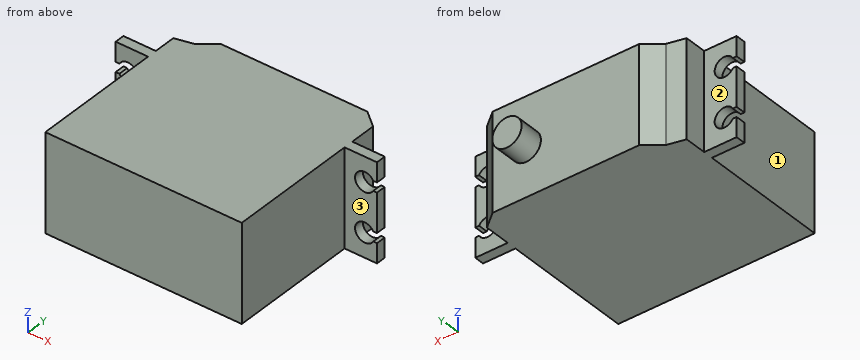
Autodesk Inventor part; units mm, degrees
ref_plane "YZ Plane" through (0, 0, 0) normal (1, 0, 0) x (0, 1, 0)
ref_plane "XZ Plane" through (0, 0, 0) normal (0, 1, 0) x (-1, 0, 0)
ref_plane "XY Plane" through (0, 0, 0) normal (0, 0, 1) x (1, 0, 0)
sketch "Skizze1" plane through (0, 0, 0) normal (0, 0, 1) x (1, 0, 0)
  line L0 (-20.15, 13.3) -> (20.15, 13.3)
  line L1 (20.15, 13.3) -> (20.15, -13.3)
  line L2 (20.15, -13.3) -> (-20.15, -13.3)
  line L3 (-20.15, -13.3) -> (-20.15, 13.3)
  line L4 (0, 30.62) -> (0, -20.62)
  line L5 (-37.52, 0) -> (37.52, 0)
  line L6 (-20.15, 13.3) -> (-20.15, 19.8141)
  line L7 (-13.1284, 23.3) -> (16.9083, 23.3)
  line L8 (20.15, 20.6722) -> (20.15, 13.3)
  line L9 (16.9083, 23.3) -> (20.15, 20.6722)
  line L10 (-20.15, 19.8141) -> (-16.5313, 20.6722)
  line L11 (-16.5313, 20.6722) -> (-13.1284, 23.3)
  line L12 (20.15, 13.3) -> (26.8, 13.3)
  line L13 (26.8, 13.3) -> (26.8, 15.3)
  line L14 (26.8, 15.3) -> (20.15, 15.3)
  line L15 (20.15, 15.3) -> (20.15, 13.3)
  line L16 (-20.15, 13.3) -> (-26.8, 13.3)
  line L17 (-26.8, 13.3) -> (-26.8, 15.3)
  line L18 (-26.8, 15.3) -> (-20.15, 15.3)
  line L19 (-20.15, 15.3) -> (-20.15, 13.3)
  line L20 (6, 23.3) -> (11, 23.3)
  point P0 (0, 0)
  dimension "d0" = 40.3
  dimension "d1" = 26.6
  dimension "d3" = 10
  dimension "d4" = 3.6187
  dimension "d5" = 3.4029
  dimension "d6" = 3.2417
  dimension "d7" = 103.34
  dimension "d8" = 142.325
  dimension "d9" = 140.972
  dimension "d10" = 6.65
  dimension "d11" = 2
  dimension "d12" = 6.65
  dimension "d13" = 2
extrude "Extrusion1" add sketch "Skizze1" along normal mid plane 20
sketch "Skizze2" plane through (-26.8, 15.3, 10) normal (0, 1, 0) x (1, 0, 0)
  line L0 (64.32, 10) -> (-10.72, 10)
  line L1 (26.8, 24) -> (26.8, -4)
  arc A0 (0.7679, 14) -> (0.7679, 16) centre (2.5, 15) ccw
  line L2 (0, 20) -> (0, 0)
  line L3 (0.7679, 16) -> (0, 16)
  line L4 (0, 20) -> (0, 0)
  line L5 (0.7679, 14) -> (0, 14)
  line L6 (0, 16) -> (0, 14)
  line L7 (2.5, 15) -> (0.8619, 15)
  arc A1 (0.7679, 4) -> (0.7679, 6) centre (2.5, 5) ccw
  line L8 (0.7679, 4) -> (0, 4)
  line L9 (0.7679, 6) -> (0, 6)
  line L10 (0, 4) -> (0, 6)
  line L11 (2.5, 5) -> (0.8619, 5)
  arc A2 (52.8321, 16) -> (52.8321, 14) centre (51.1, 15) ccw
  line L12 (52.8321, 16) -> (53.6, 16)
  line L13 (52.8321, 14) -> (53.6, 14)
  line L14 (53.6, 16) -> (53.6, 14)
  line L15 (51.1, 15) -> (52.7381, 15)
  arc A3 (52.8321, 6) -> (52.8321, 4) centre (51.1, 5) ccw
  line L16 (52.8321, 4) -> (53.6, 4)
  line L17 (52.8321, 6) -> (53.6, 6)
  line L18 (53.6, 4) -> (53.6, 6)
  line L19 (51.1, 5) -> (52.7381, 5)
  point P0 (26.8, 10)
  dimension "d19" = 4
  dimension "d21" = 5
  dimension "d23" = 2.5
  dimension "d25" = 2
extrude "Extrusion2" cut sketch "Skizze2" against normal up to surface (2 mm away)
sketch "Skizze3" plane through (-13.1284, 23.3, 10) normal (0, 1, 0) x (1, 0, 0)
  line L0 (13.1284, 24) -> (13.1284, -4)
  line L1 (-24.3916, 10) -> (50.6484, 10)
  circle A0 centre (23.1284, 10) radius 3
  point P0 (13.1284, 10)
  dimension "d28" = 6
  dimension "d29" = 10
extrude "Extrusion3" add sketch "Skizze3" along normal blind 5
properties part number "Servo"
For this review, take the finished solid that the model builds, in its own axes (mm). Face numbers are marked on the shaded views. A direction names the side the tool comes from. Coordinates: 2 decimals unless noted, no trailing zeros. Loops run counter-clockwise (first coordinate to the right, second up) from the corner with the lowest first, then second, coordinate; pieces in that order, holes last. Notation, with made-up numbers: (-36.75, -13.75) - (-3.75, -13.75) arc R25 ccw to (-3.75, 10.25) - close; hole circle Ø8 at (48, -21). An arc over 180 degrees is marked (long way). Use one line per item in the form item = value. Start each with the question number.
1) To check wall thickness, follow probe 1 along Z at (x, y) = (-24, 14); probe 2 along Y at (x, z) = (-8, 0.25); probe 3 along X at (y, z) = (7, 3.75). State the ranges of each line that lie inside material, in increasing order. Write a range as from..to.
2) Take a section at B-B (y = 14.5). State the section outline as (x, z) points.
3) Take a section at A-A (x = -24.3). State the section outline as (y, z) points, plus the area to 3 significant figures.
4) Take a section at D-D (z = 0). State the section outline as (x, y) points.
5) For pin 1 (5 mm diameter, centred on x = 24.3, z = -5, fed in from -Y); pin 2 (5 mm diameter, centred on y = 20, z = -4.5, fed in from -X); pin 3 (2.5 mm diameter, centred on x = -24.3, z = 5, fed in from -Y); pin 4 (5 mm diameter, centred on x = 0, z = 3.5, fed in from +Y), all flat-tipped, find the tip position at first contact; note any pin that passes through.
6) Take a section at C-C (x = 10). State the section outline as (y, z) points, plus the area to 3 significant figures.
7) For the marked faces 1, 2 and 3, list the 3-axis set-ups (+Z, -Z, +X, -X, +Y, -Y) from which the entire face can be reached by the end or side of a thin tool; tool diameter is ignored.
From the geometry:
q1.probe_1 = -10..-6.98, -3.02..3.02, 6.98..10
q1.probe_2 = -13.3..23.3
q1.probe_3 = -20.15..20.15
q2.outline = (-26.8, -10) - (26.8, -10) - (26.8, -6) - (26.03, -6) arc R2 cw (long way) to (26.03, -4) - (26.8, -4) - (26.8, 4) - (26.03, 4) arc R2 cw (long way) to (26.03, 6) - (26.8, 6) - (26.8, 10) - (-26.8, 10) - (-26.8, 6) - (-26.03, 6) arc R2 cw (long way) to (-26.03, 4) - (-26.8, 4) - (-26.8, -4) - (-26.03, -4) arc R2 cw (long way) to (-26.03, -6) - (-26.8, -6) - close
q3.outline = (13.3, -10) - (15.3, -10) - (15.3, -7) - (13.3, -7) - close; (13.3, -3) - (15.3, -3) - (15.3, 3) - (13.3, 3) - close; (13.3, 7) - (15.3, 7) - (15.3, 10) - (13.3, 10) - close
q3.area = 24.0 mm2
q4.outline = (-26.8, 13.3) - (-20.15, 13.3) - (-20.15, -13.3) - (20.15, -13.3) - (20.15, 13.3) - (26.8, 13.3) - (26.8, 15.3) - (20.15, 15.3) - (20.15, 20.67) - (16.91, 23.3) - (13, 23.3) - (13, 28.3) - (7, 28.3) - (7, 23.3) - (-13.13, 23.3) - (-16.53, 20.67) - (-20.15, 19.81) - (-20.15, 15.3) - (-26.8, 15.3) - close
q5.pin_1 = 13.3
q5.pin_2 = -20.15
q5.pin_3 = through
q5.pin_4 = 23.3
q6.outline = (-13.3, -10) - (23.3, -10) - (23.3, -3) - (28.3, -3) - (28.3, 3) - (23.3, 3) - (23.3, 10) - (-13.3, 10) - close
q6.area = 762 mm2
q7.face_1 = +Z, -Z, -X, -Y
q7.face_2 = +Z, -Z, -X, +Y
q7.face_3 = +Z, -Z, +X, -Y
